Verification items for this drawing (mm, ordinates from the low corner). A direction names the side the tool comes from. Give positions to 0.01 mm unless a question says otherwise; leave off trailing zeros. Order: outer loops, then holes, each group sorted by start corner. A loop starts at its lowest first (then second) coordinate and runs counter-clockwise, first axis right, second up.
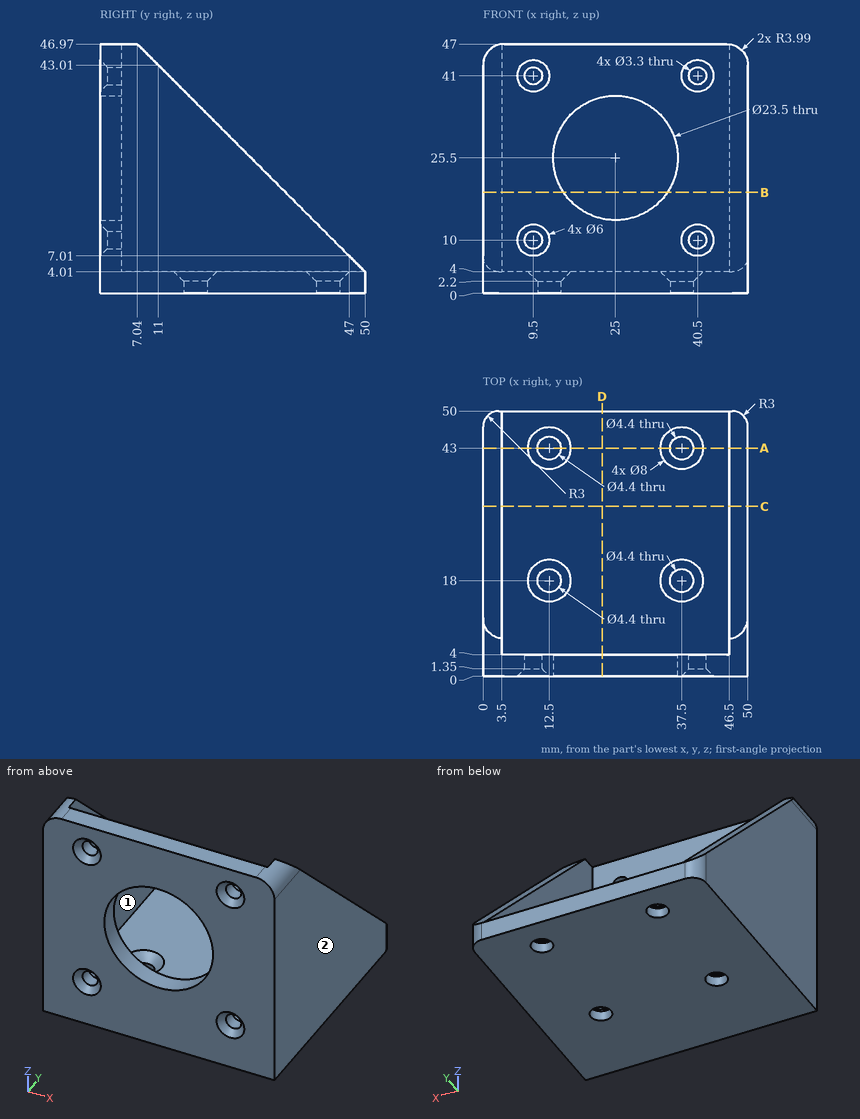
Q1. Thickness scan on L1, parallel to X at y = 18, z = 1.05; L2, parallel to Z at x = 40.5, y = 2.5; L3, parallel to Y at x = 37.5, z = 1.55. Record the ranges inside material, lowest first.
Q2. Cross-section at B-B, the plane z = 19. Record the boundary of the cut face in (x, y), and give its area (3 significant figures).
Q3. Cross-section at A-A, the plane y = 43. Record the boundary of the cut face in (x, z).
Q4. Cross-section at D-D, the plane x = 22.5. Record the boundary of the cut face in (y, z), and give its area (3 significant figures).
Q5. Access from +Z, -Z, +X, -X, +Y, -Y to the whole of each face (thin tool, end or side, straight path). Record for the marked faces 1 and 2.
Q6. Gauge pin test, flat ends, axial feed: P1, Ø5.5, axis at x = 9.5, z = 10, coming from the +Y side; P2, Ø7, axis at x = 37.5, y = 43, coming from the +Z side; P3, Ø4.5, axis at x = 40.5, z = 41, coming from the -Y side. Record the tip position at first contact, or that the pin passes through.
Q7. Cross-section at C-C, the plane y = 32. Record the boundary of the cut face in (x, z).
Answers follow:
1. L1: x = 0 to 10.3, 14.7 to 35.3, 39.7 to 50
1. L2: z = 0 to 8.35, 11.65 to 39.35, 42.65 to 47
1. L3: y = 0 to 15.8, 20.2 to 40.8, 45.2 to 50
2. outline: (0, 0) - (15.21, 0) - (15.21, 4) - (3.5, 4) - (3.5, 35.01) - (0, 35.01) - close; (34.79, 0) - (50, 0) - (50, 35.01) - (46.5, 35.01) - (46.5, 4) - (34.79, 4) - close
2. area: 339 mm2
3. outline: (0, 0) - (10.3, 0) - (10.3, 2.2) - (8.5, 4) - (3.5, 4) - (3.5, 11.01) - (0, 11.01) - close; (14.7, 0) - (35.3, 0) - (35.3, 2.2) - (33.5, 4) - (16.5, 4) - (14.7, 2.2) - close; (39.7, 0) - (50, 0) - (50, 11.01) - (46.5, 11.01) - (46.5, 4) - (41.5, 4) - (39.7, 2.2) - close
4. outline: (0, 0) - (50, 0) - (50, 4) - (4, 4) - (4, 14.02) - (0, 14.02) - close; (0, 36.98) - (4, 36.98) - (4, 47) - (0, 47) - close
4. area: 280 mm2
5. face 1: +Z, +Y
5. face 2: +Z, -Z, +X, +Y, -Y
6. P1: stops at y = 4
6. P2: stops at z = 3.5
6. P3: stops at y = 0.75
7. outline: (0, 0) - (50, 0) - (50, 22.01) - (46.5, 22.01) - (46.5, 4) - (3.5, 4) - (3.5, 22.01) - (0, 22.01) - close
